Verification items for the finished model (mm, model axes). Coordinates: 2 decimals unless noted, no trailing zeros. Order: outer loops, then holes, each group sorted by start corner. A loop starts at its lowest first (then second) coordinate and runs counter-clockwise, first axis right, second up. Notation, with made-up numbers: M 36,18 L 80,18 A24 cw 80,32 Z; hole C 45.25,-21.5 d6. An arc over 180 degrees is marked long. Return JSON: item names as keys, results as strings. Group by question number.
Q1. Thickness scan on probe 1 along X at (y, z) = (424.5, 2.5); probe 2 along X at (y, z) = (548, 1); probe 3 along Z at (x, y) = (121.5, 900). Record the ranges inside material, lowest first.
Q2. Go/stop test with flat-tipped pins: pin 1 Ø5 at (x, z) = (397.5, 3) entering from -Y; pin 2 Ø5 at (x, z) = (172.5, 2.5) entering from -Y; pin 3 Ø12 at (y, z) = (752.5, 19) entering from +X. Record where each tip stops, or that it passes through.
Q3. Section check A-A, the plane y = 680.5. Enter the section's corners in (x, z), then the cut area to 3 significant figures.
Q4. Section check B-B, the plane x = 0. Enter the section's corners in (y, z), then the cut area to 3 significant figures.
Q5. Section check C-C, the plane y = 815. Enter the section's corners in (x, z).
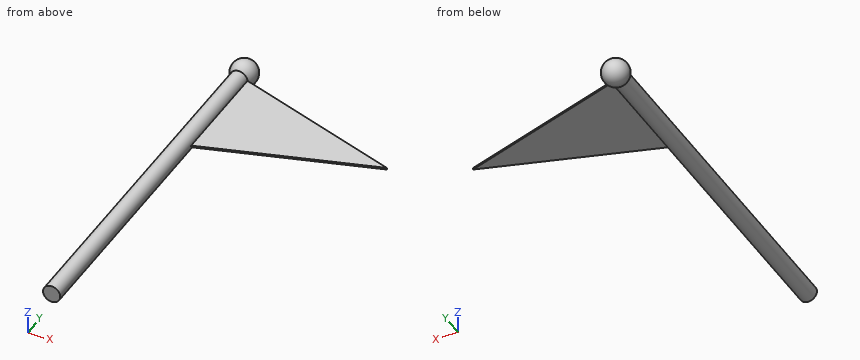
from build123d import *

# Parameters (mm, degrees)
SKETCH1_R           = 24.5
BOSS_EXTRUDE1_DEPTH = 1000
BOSS_EXTRUDE2_DEPTH = 2.5


with BuildPart() as part:
    # Sketch1 → Boss-Extrude1 (new body)
    with BuildSketch(Plane(origin=(0, 0, 0), x_dir=(1, 0, 0), z_dir=(0, 1, 0))):
        Circle(SKETCH1_R)
    extrude(amount=BOSS_EXTRUDE1_DEPTH)

    # Sketch2 → Revolve5 (revolve)
    with BuildSketch(Plane.XY):
        with BuildLine():
            Line((0, 1062.5), (0, 987.5))
            ThreePointArc((0, 987.5), (37.5, 1025), (0, 1062.5))
        make_face()
    revolve(axis=Axis((0, 1062.5, 0), (0, -1, 0)))

    # Sketch3 → Boss-Extrude2 (add, symmetric)
    with BuildSketch(Plane.XY):
        Polygon((24.5, 996.609860867), (500, 846.609860867), (24.5, 696.609860867), (0, 696.609860867), (0, 996.609860867), align=None)
    extrude(amount=BOSS_EXTRUDE2_DEPTH, both=True)


solid = part.part
Numbers:
{
 "1": {"probe 1": "x = -24.37 to 24.37", "probe 2": "x = -24.48 to 24.48", "probe 3": "z = -2.5 to 2.5"},
 "2": {"pin 1": "stops at y = 813.5", "pin 2": "stops at y = 742.51", "pin 3": "stops at x = 20.77"},
 "3": {"outline": "C 0,0 d49", "area": "1,890 mm2"},
 "4": {"outline": "M 0,-24.5 L 996.61,-24.5 A37.5 ccw long 996.61,24.5 L 0,24.5 Z", "area": "52,900 mm2"},
 "5": {"outline": "M 24.37,-2.5 L 399.8,-2.5 L 399.8,2.5 L 24.37,2.5 A24.5 ccw long Z"}
}
